Design review of the part shown in the three views and the two pictorial views. Dimensions are in mm from the part's minimum x, y and z. A direction names the side the tool comes from. Give positions to 0.01 mm unless a question says otherwise; leave off trailing zeros. Loops run counter-clockwise (first coordinate to the right, second up) from the corner with the lowest first, then second, coordinate; pieces in that order, holes last. Notation, with made-up numbers: (-24, -3) -> (25, -3) arc R14 ccw to (25, 19) -> close; hole circle Ø1 at (72, -15). An arc over 180 degrees is marked (long way). Answer as CSV lines item,"result". Start each with the question number.
Item 1: Machinability: for the marked faces 4, 5 and 6, which of the approach directions +Z, -Z, +X, -X, +Y, -Y give a long, thin tool a straight path to every point of the face, cutting with its end or side? Answer none if there is none.
Item 2: Clearance check with flat-ended pins moving along their axes: P1, Ø8, axis at x = 30, y = 55, coming from the +Z side; P2, Ø1.5, axis at x = 7.5, y = 34.5, coming from the -Z side; P3, Ø10, axis at x = 37, z = 23, coming from the -Y side; P4, Ø1.5, axis at x = 18.5, z = 32, coming from the -Y side. State where each tip first meets the part, or that it passes through.
Item 3: Add section A-A on z = 32. State the section outline as (x, y) points.
Item 4: The part is to be moulded in two halves that separate along Y. For the marked faces 1, 2 and 3, say which applies: +Y half, -Y half, draft (parallel to the pull), parting line (faces both ways), or undercut.
Item 5: For L1, parallel to Y at x = 30, z = 48; L2, parallel to X at y = 17, z = 48; L3, parallel to Y at x = 41, z = 8, list the stretches that pass through material, from the lowest coordinate up. Write a range as from..to.
Item 6: Add section D-D on y = 55. State the section outline as (x, z) points.
Item 7: Add section B-B on y = 17.5. State how many separate pieces and enclosed holes the cut face has, plus the area to 3 significant figures.
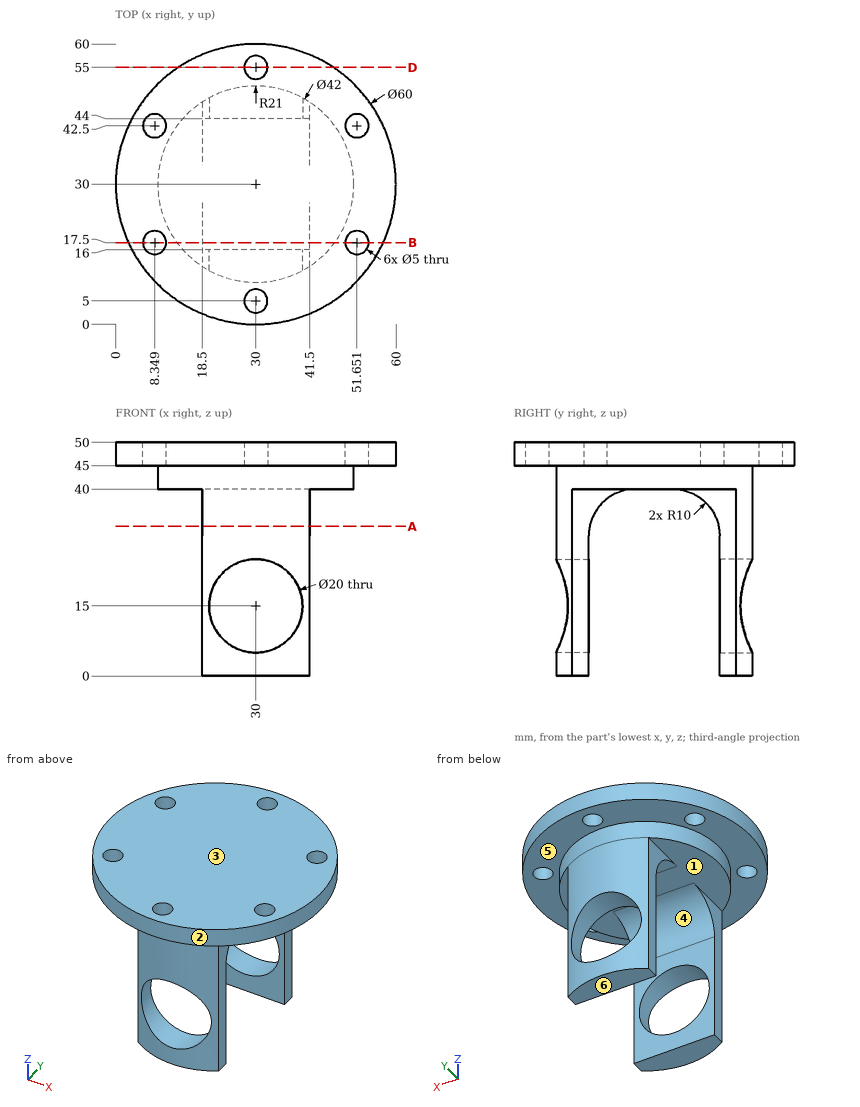
Computed values:
1,face 4,"-Z, +X, -X"
1,face 5,"-Z"
1,face 6,"-Z, +X, -X, +Y, -Y"
2,P1,"z = 50"
2,P2,"z = 45"
2,P3,"y = 9.13"
2,P4,"y = 11.96"
3,outline,"(18.5, 12.43) arc R21 ccw to (41.5, 12.43) -> (41.5, 16.2) -> (18.5, 16.2) -> close; (18.5, 43.8) -> (41.5, 43.8) -> (41.5, 47.57) arc R21 ccw to (18.5, 47.57) -> close"
4,face 1,"undercut"
4,face 2,"parting line"
4,face 3,"draft"
5,L1,"0..2.5, 7.5..52.5, 57.5..60"
5,L2,"2.96..5.9, 10.8..49.2, 54.1..57.04"
5,L3,"12.11..16, 44..47.89"
6,outline,"(13.42, 45) -> (27.5, 45) -> (27.5, 50) -> (13.42, 50) -> close; (32.5, 45) -> (46.58, 45) -> (46.58, 50) -> (32.5, 50) -> close"
7,separate pieces,"3"
7,enclosed holes,"0"
7,area,"500 mm²"
